Autodesk Inventor part; units mm, degrees
ref_plane "YZ Plane" through (0, 0, 0) normal (1, 0, 0) x (0, 1, 0)
ref_plane "XZ Plane" through (0, 0, 0) normal (0, 1, 0) x (-1, 0, 0)
ref_plane "XY Plane" through (0, 0, 0) normal (0, 0, 1) x (1, 0, 0)
sketch "Sketch1" plane through (0, 0, 0) normal (0, 0, 1) x (1, 0, 0)
  circle A0 centre (0, 0) radius 6.2865
  circle A1 centre (0, 0) radius 7.7343
  circle A2 centre (0, 0) radius 12.7
  dimension "d0" = 12.573
  dimension "d1" = 15.4686
  dimension "d4" = 25.4
extrude "Extrusion2" add sketch "Sketch1" along normal blind 100 contours A1 | A2
extrude "Extrusion3" cut sketch "Sketch1" along normal blind 10.0076 contours A2
sketch "Sketch3" plane through (0, 0, 100) normal (0, 0, 1) x (1, 0, 0)
  circle A0 centre (0, 0) radius 12.7
  circle A1 centre (0, 0) radius 7.7343
  circle A2 centre (0, 0) radius 6.2865
  circle A3 centre (0, 0) radius 6.2865
  circle A4 centre (0, 0) radius 6.2865
extrude "Extrusion4" cut sketch "Sketch3" against normal blind 85.598 contours A0
sketch "Sketch4" plane through (0, 0, 10.0076) normal (0, 0, -1) x (-1, 0, 0)
  circle A0 centre (0, 0) radius 10.6045 construction
  point P0 (0, 10.6045)
  point P1 (0, -10.6045)
  point P2 (-10.6045, 0)
  point P3 (10.6045, 0)
  dimension "d11" = 21.209
hole "Hole1" at (0, 10.6045, 10.0076) at (10.6045, 0, 10.0076) at (-10.6045, 0, 10.0076) at (0, -10.6045, 10.0076) direction (0, 0, 1) diameter 1.5748 depth 6.2992 tip angle 118
sketch "Sketch5" plane through (0, 0, 10.0076) normal (0, 0, -1) x (-1, 0, 0)
  point P0 (0, 0)
sketch "Sketch6" plane through (0, 0, 10.0076) normal (0, 0, -1) x (-1, 0, 0)
  circle A0 centre (0, 10.6045) radius 0.7874 construction
  line L0 (0, 10.6045) -> (0, 12.7) construction
  circle A1 centre (0, 0) radius 12.7 construction
properties part number "waveguide"
The model under review builds one solid part; all positions refer to its coordinate system, in mm. A direction names the side the tool comes from. Round coordinates to 2 decimals unless told otherwise and drop trailing zeros. Loops run counter-clockwise (first coordinate to the right, second up) from the corner with the lowest first, then second, coordinate; pieces in that order, holes last. Notation, with made-up numbers: (-8.5, 89.5) - (31.5, 89.5) arc R16 cw to (31.5, 107.5) - close; hole circle Ø4 at (49, 23.5). An arc over 180 degrees is marked (long way). Write each question's results on one line, items separated by ' | '. Start each with the question number.
Q1. Take a section at A-A on x = 3.25. Give the boundary of the cut face in (y, z).
Q2. Insertion check: P1, Ø1.5, axis at x = 7.5, z = 15.5, coming from the +Y side; P2, Ø8, axis at y = 4, z = 81.5, coming from the +X side; P3, Ø4, axis at x = -4, z = 48, coming from the -Y side. Each pin has a flat end and moves straight along its axis. Give the tip position at first contact, or say it passes through.
Q3. Draft analysis for pull direction X (two halves, no side actions). For faces 4 (the cylindrical face through (-1.363, 6.137, 49.3)), 5 (the cylindrical face through (-6.138, 4.706, 4.934)), 6 (the flat face through (-5.8, -5.5, 14.402)), state which applies: pulls with the +X half, pulls with the -X half, needs draft (parallel to the pull), parting line crosses it, or undercut.
Q4. Tool access review of faces 1 (the cylindrical face through (-2.75, 12.4, 12.17)), 2 (the cylindrical face through (-6.138, -4.706, 57.8)), 3 (the flat face through (-5.8, -5.5, 10.008)): name each direction out of +Z, -Z, +X, -X, +Y, -Y from which nothing blocks a thin tool from reaching the whole face with its end or side.
Q5. Wall thickness on line 1 along Y through (x, z) = (0, 11.3); line 2 along Y through (x, z) = (0.25, 88.5); line 3 along X through (y, z) = (2.25, 74.5): over which ranges is each line inside the solid? List them lowest first. Write a range as [from, to].
Q6. Take a section at B-B on z = 36. Give the boundary of the cut face in (x, y), plus the area to 3 significant figures.
Q7. Take a section at C-C on y = -3.5. Give the boundary of the cut face in (x, z), plus the area to 3 significant figures.
Data:
1) outline: (-12.28, 10.01) - (-7.02, 10.01) - (-7.02, 0) - (-5.38, 0) - (-5.38, 100) - (-7.02, 100) - (-7.02, 14.4) - (-12.28, 14.4) - close; (5.38, 0) - (7.02, 0) - (7.02, 10.01) - (12.28, 10.01) - (12.28, 14.4) - (7.02, 14.4) - (7.02, 100) - (5.38, 100) - close
2) P1: stops at y = 3.78 | P2: stops at x = 7.73 | P3: stops at y = -7.47
3) face 4: undercut | face 5: parting line crosses it | face 6: needs draft
4) face 1: +Z, -Z | face 2: +Z | face 3: -Z
5) line 1: y = [-12.7, -11.39], [-9.82, -6.29], [6.29, 9.82], [11.39, 12.7] | line 2: y = [-7.73, -6.28], [6.28, 7.73] | line 3: x = [-7.4, -5.87], [5.87, 7.4]
6) outline: circle Ø15.47 at (0, 0); hole circle Ø12.57 at (0, 0) | area: 63.8 mm²
7) outline: (-12.21, 10.01) - (-6.9, 10.01) - (-6.9, 0) - (-5.22, 0) - (-5.22, 100) - (-6.9, 100) - (-6.9, 14.4) - (-12.21, 14.4) - close; (5.22, 0) - (6.9, 0) - (6.9, 10.01) - (12.21, 10.01) - (12.21, 14.4) - (6.9, 14.4) - (6.9, 100) - (5.22, 100) - close | area: 382 mm²
